Input: part model. Units: mm. Frame: model coordinates. A direction names the side the tool comes from. Coordinates: 2 decimals unless noted, no trailing zeros. Order: outer loops, then holes, each group sorted by start corner. A loop starts at its lowest first (then second) coordinate and runs counter-clockwise, first axis right, second up. Notation, with made-up numbers: (-25, -21.5) -> (5, -21.5) arc R22 ccw to (5, 14.5) -> close; hole circle Ø1 at (-8.5, 20). An arc over 180 degrees is marked (long way). Use one line per item in the form item = value. Start each with the question number.
1) Pin query (flat end, axial travel): pin 1 (5 mm diameter, centred on x = -63.5, z = -9.5, fed in from -Y); pin 2 (4 mm diameter, centred on y = -26, z = -2.5, fed in from -X); pin 3 (6 mm diameter, centred on x = 80, z = 0.5, fed in from -Y) (3 decimals). Return the tip coordinate at first contact, or that it passes through.
2) Access query for faces 1 (the flat face through (-215.9, 0, 0)), 2 (the cylindrical face through (390.54, -166.34, 0.7)). Directions: +Z, -Z, +X, -X, +Y, -Y. A direction counts if a zero-diameter tool reaches every point of the face in a straight line with its end or side. Return the directions, or none.
3) Section query C-C on y = -131.5. Output: boundary loops of the cut face in (x, z) (3 decimals).
4) Section query A-A on z = 0. Output: boundary loops of the cut face in (x, y) (3 decimals), then the cut area to 3 significant figures.
5) Ray query, line 1 along X through (y, z) = (-93, -0.5); line 2 along X through (y, z) = (-180, -14); line 3 along Y through (x, z) = (198.5, -6). Return the intervals inside material, ascending.
6) Section query B-B on x = 173. Output: boundary loops of the cut face in (y, z) (3 decimals).
from build123d import *

# Parameters (mm, degrees)
F2_R     = 15.875
F4_R     = 3.175
F5_DEPTH = 22.225
F6_R     = 15.875
F7_DEPTH = 63.5


with BuildPart() as f3:
    # F3: sweep along a path in F0
    with BuildLine(Plane.XY) as f3_path:
        Line((-152.4, 0), (0, 0))
        Line((0, 0), (330.2, 0))
        ThreePointArc((330.2, 0), (384.0815367264, -22.3184632736), (406.4, -76.2))
        Line((406.4, -76.2), (406.4, -254))
    # F2 (on offset) → F3 (sweep)
    with BuildSketch(Plane.XZ.offset(254)):
        with Locations((406.4, 0)):
            Circle(F2_R)
    sweep(path=f3_path.line)

    # F4 (on Top) → F5 (join)
    with BuildSketch(Plane.XY):
        with Locations((-50.8, 0)):
            Circle(F4_R)
    extrude(amount=F5_DEPTH)

    # F6 (on face) → F7 (join)
    with BuildSketch(Plane(origin=(-152.4, 0, 0), x_dir=(0, -1, 0), z_dir=(-1, 0, 0))):
        Circle(F6_R)
    extrude(amount=F7_DEPTH)


solid = f3.part
Answers below:
q1.pin_1 = -14.25
q1.pin_2 = 360.78
q1.pin_3 = -15.875
q2.face_1 = +Z, -Z, -X, +Y, -Y
q2.face_2 = -Y
q3.outline = circle Ø31.75 at (406.4, 0)
q4.outline = (-215.9, -15.875) -> (330.2, -15.875) arc R60.325 cw to (390.525, -76.2) -> (390.525, -254) -> (422.275, -254) -> (422.275, -76.2) arc R92.075 ccw to (330.2, 15.875) -> (-215.9, 15.875) -> close
q4.area = 26,800 mm^2
q5.line_1 = 390.53 to 422.27
q5.line_2 = 398.92 to 413.88
q5.line_3 = -14.7 to 14.7
q6.outline = circle Ø31.75 at (0, 0)
